Could you check a few things on this drawing? It's one solid part, dimensions in mm from its lowest x, y, z. A direction names the side the tool comes from. Give positions to 0.01 mm unless a question says otherwise; leave off trailing zeros. Order: outer loops, then holes, each group sorted by start corner. A loop starts at its lowest first (then second) coordinate and runs counter-clockwise, first axis right, second up. Notation, with made-up numbers: (44.5, 19) - (67.5, 19) arc R17 cw to (67.5, 42) - close; hole circle Ø5 at (53, 0). An arc over 180 degrees is marked (long way). Put each result on its own line as item: value.
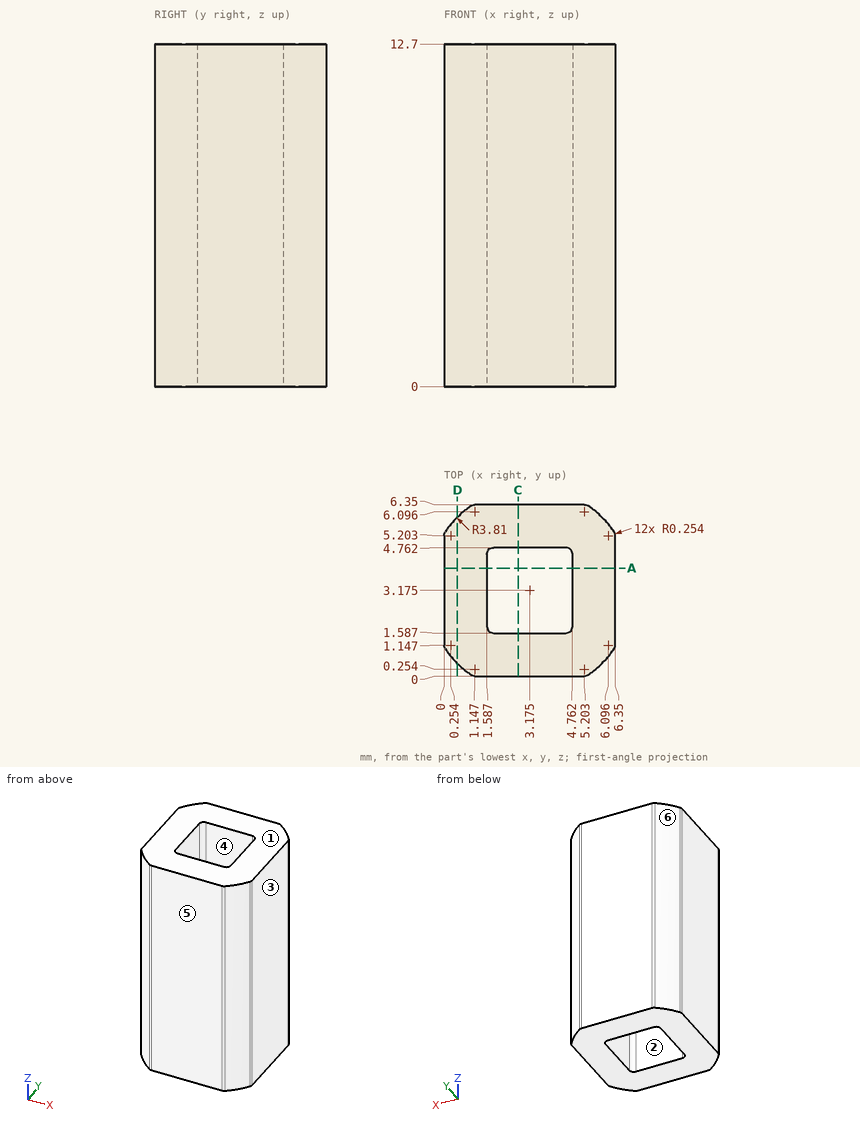
1) Suppose I cut it at A-A, the plane y = 4. List the corners of the cut face in (x, z) for me.
Filled in:
outline: (0, 0) - (1.59, 0) - (1.59, 12.7) - (0, 12.7) - close; (4.76, 0) - (6.35, 0) - (6.35, 12.7) - (4.76, 12.7) - close
2) We'd pull the mould along X, two halves only. Please class the marked faces 3, 4, 5 and 6: pulls with the +X half, pulls with the -X half, needs draft (parallel to the pull), parting line crosses it, or undercut.
Filled in:
face 3: pulls with the +X half
face 4: undercut
face 5: needs draft
face 6: pulls with the -X half
3) Suppose I cut it at D-D, the plane x = 0.5. List the corners of the cut face in (y, z) for me.
Filled in:
outline: (0.46, 0) - (5.89, 0) - (5.89, 12.7) - (0.46, 12.7) - close
4) Which directions (+Z, -Z, +X, -X, +Y, -Y) give clear straight access to the entire face, cutting with the end or side of a thin tool? Please do the marked faces 1 and 2.
Filled in:
face 1: +Z, +X, -X, +Y, -Y
face 2: +Z, -Z
5) If I drill on line 1 (Y direction, x = 4.5, z = 2.25); line 2 (X direction, y = 1, z = 5.5) (1 decimal), over which ranges is the centre line in solid material (lowest first)? Write a range as [from, to].
Filled in:
line 1: y = [0, 1.59], [4.76, 6.35]
line 2: x = [0, 6.3]
